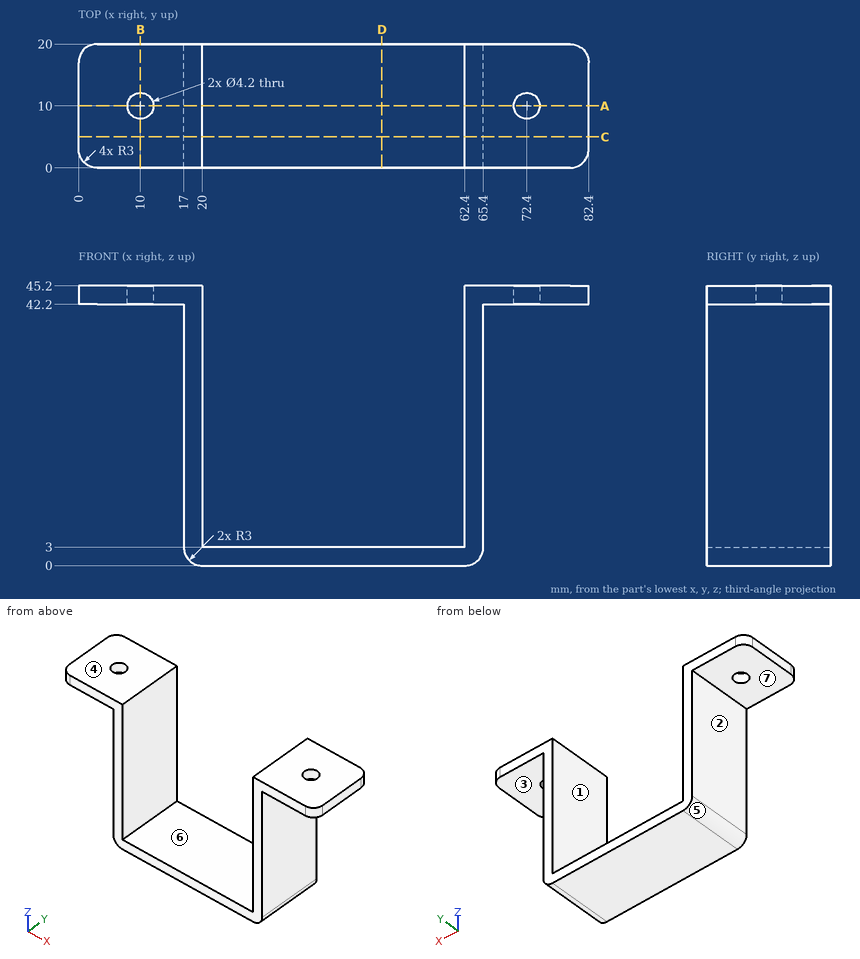
Input: dimensioned drawing with shaded views. Units: mm. Origin: part minimum x, y, z. A direction names the side the tool comes from. Give positions to 0.01 mm unless a question says otherwise; leave off trailing zeros. Write each loop counter-clockwise with the first axis right and the second up, starting at its lowest first coordinate (ties: lowest second). Pieces come first, ordered by that corner, then holes. Notation, with made-up numbers: (63.5, -5) -> (95.5, -5) arc R15 ccw to (95.5, 4) -> close; hole circle Ø8 at (3.25, 83.25). An arc over 180 degrees is marked (long way). Answer as a JSON object with one key per item and string values.
1. Cut plane B-B on x = 10. Output: boundary loops of the cut face in (y, z).
Ans:
{"outline": "(0, 42.2) -> (7.9, 42.2) -> (7.9, 45.2) -> (0, 45.2) -> close; (12.1, 42.2) -> (20, 42.2) -> (20, 45.2) -> (12.1, 45.2) -> close"}
2. Ray query, probe 1 along Y at (x, z) = (72.4, 44.3); probe 2 along X at (y, z) = (15, 35.5); probe 3 along Z at (x, y) = (65.5, 5). Return the intervals inside material, ascending. Write a range as from..to.
Ans:
{"probe 1": "y = 0..7.9, 12.1..20", "probe 2": "x = 17..20, 62.4..65.4", "probe 3": "z = 42.2..45.2"}
3. Cut plane D-D on x = 49. Output: boundary loops of the cut face in (y, z).
Ans:
{"outline": "(0, 0) -> (20, 0) -> (20, 3) -> (0, 3) -> close"}
4. Mould query, pull axis X, two halves, no side actions, for the marked faces 5, 6 and 7. Classes: pulls with the +X half, pulls with the -X half, needs draft (parallel to the pull), parting line crosses it, or undercut.
Ans:
{"face 5": "pulls with the -X half", "face 6": "undercut", "face 7": "needs draft"}
5. Contact query for flat-ended pins moving along their axis: pin 1 (10 mm diameter, centred on x = 31, y = 6.5, fed in from +Z); pin 2 (2 mm diameter, centred on y = 12.5, z = 18.5, fed in from -X); pin 3 (8.5 mm diameter, centred on x = 12.5, y = 10, fed in from -Z). Output: stop coordinate, or through.
Ans:
{"pin 1": "stops at z = 3", "pin 2": "stops at x = 17", "pin 3": "stops at z = 42.2"}
6. Cut plane A-A on y = 10. Output: boundary loops of the cut face in (x, z).
Ans:
{"outline": "(0, 42.2) -> (7.9, 42.2) -> (7.9, 45.2) -> (0, 45.2) -> close; (12.1, 42.2) -> (17, 42.2) -> (17, 3) arc R3 ccw to (20, 0) -> (62.4, 0) arc R3 ccw to (65.4, 3) -> (65.4, 42.2) -> (70.3, 42.2) -> (70.3, 45.2) -> (62.4, 45.2) -> (62.4, 3) -> (20, 3) -> (20, 45.2) -> (12.1, 45.2) -> close; (74.5, 42.2) -> (82.4, 42.2) -> (82.4, 45.2) -> (74.5, 45.2) -> close"}
7. Cut plane C-C on y = 5. Output: boundary loops of the cut face in (x, z), and give its area (3 significant figures).
Ans:
{"outline": "(0, 42.2) -> (17, 42.2) -> (17, 3) arc R3 ccw to (20, 0) -> (62.4, 0) arc R3 ccw to (65.4, 3) -> (65.4, 42.2) -> (82.4, 42.2) -> (82.4, 45.2) -> (62.4, 45.2) -> (62.4, 3) -> (20, 3) -> (20, 45.2) -> (0, 45.2) -> close", "area": "497 mm^2"}
8. Access query for the marked faces 1, 2, 3 and 4. Directions: +Z, -Z, +X, -X, +Y, -Y. A direction counts if a zero-diameter tool reaches every point of the face in a straight line with its end or side. Return the directions, or none.
Ans:
{"face 1": "+Z, +Y, -Y", "face 2": "-Z, -X, +Y, -Y", "face 3": "-Z, +X, +Y, -Y", "face 4": "+Z, +X, -X, +Y, -Y"}
